from build123d import *

# Parameters (mm, degrees)
F0_W     = 685.8
F0_H     = 101.6
F1_DEPTH = 19.05
F2_W     = 222.25
F2_H     = 14.1
F3_DEPTH = 10.16
F4_R     = 3.302
F5_DEPTH = 25.4


with BuildPart() as f1:
    # F0 (on Front) → F1 (new body)
    with BuildSketch(Plane.XZ):
        with Locations((45.375204, 0)):
            Rectangle(F0_W, F0_H)
    extrude(amount=F1_DEPTH)

    # F2 (on face) → F3 (cut)
    with BuildSketch(Plane(origin=(0, 0, 0), x_dir=(-1, 0, 0), z_dir=(0, 1, 0))):
        with Locations((-258.100204, 0)):
            Rectangle(F2_W, F2_H)
    extrude(amount=-F3_DEPTH, mode=Mode.SUBTRACT)

    # F4 (on face) → F5 (cut)
    with BuildSketch(Plane.XZ.offset(19.05)):
        with BuildLine():
            ThreePointArc((382.052204, 0), (381.085071, 2.334867), (378.750204, 3.302))
            Line((378.750204, 3.302), (378.750204, 0))
            Line((378.750204, 0), (378.750204, -3.302))
            ThreePointArc((378.750204, -3.302), (381.085071, -2.334867), (382.052204, 0))
        make_face()
        with BuildLine():
            Line((378.750204, 0), (378.750204, 3.302))
            ThreePointArc((378.750204, 3.302), (375.448204, 0), (378.750204, -3.302))
            Line((378.750204, -3.302), (378.750204, 0))
        make_face()
        with Locations((137.450204, 0)):
            Circle(F4_R)
        with Locations((-287.999796, 0)):
            Circle(F4_R)
    extrude(amount=-F5_DEPTH, mode=Mode.SUBTRACT)


solid = f1.part
Verification items for the finished model (mm, model axes). Coordinates: 2 decimals unless noted, no trailing zeros. Loops run counter-clockwise (first coordinate to the right, second up) from the corner with the lowest first, then second, coordinate; pieces in that order, holes last. Notation, with made-up numbers: (22.5, 30.25) -> (65.5, 30.25) arc R15 ccw to (65.5, 39.25) -> close; hole circle Ø10 at (2, 67). An arc over 180 degrees is marked (long way). Answer as CSV lines item,"result".
1) Thickness scan on L1, parallel to X at y = -1.25, z = 7; L2, parallel to Z at x = 247.5, y = -5.75; L3, parallel to Y at x = 330, z = -6. Record the ranges inside material, lowest first. Write a range as from..to.
Found:
L1,"x = -297.52..146.98, 369.23..388.28"
L2,"z = -50.8..-7.05, 7.05..50.8"
L3,"y = -19.05..-10.16"
2) Depth check by flat-ended pin: pin 1 (3 mm diameter, centred on x = -108.5, z = -24, fed in from +Y); pin 2 (6 mm diameter, centred on x = 137.45, z = 0, fed in from -Y). Enter the tip coordinate at first touch or a pass-through.
Found:
pin 1,"stops at y = 0"
pin 2,"passes through"
3) Cross-section at B-B, the plane x = 175. Record the cut outline in (y, z), then the cut area to 3 significant figures.
Found:
outline,"(-19.05, -50.8) -> (0, -50.8) -> (0, -7.05) -> (-10.16, -7.05) -> (-10.16, 7.05) -> (0, 7.05) -> (0, 50.8) -> (-19.05, 50.8) -> close"
area,"1,790 mm2"
4) Release check for a two-part mould opening along Z. For faces 1 (the flat face through (260, -10.16, 0)), 2 (the flat face through (41, -9, 50.8)), 3 (the flat face through (41, -9, -50.8)), 4 (the flat face through (41, -19.05, 1)) record: +Z half, -Z half, draft (parallel to the pull), parting line (faces both ways), or undercut.
Found:
face 1,"undercut"
face 2,"+Z half"
face 3,"-Z half"
face 4,"draft"
5) Cross-section at A-A, the plane y = -6.25. Record the cut outline in (x, z).
Found:
outline,"(-297.52, -50.8) -> (388.28, -50.8) -> (388.28, 50.8) -> (-297.52, 50.8) -> close; hole circle Ø6.6 at (-288, 0); hole circle Ø6.6 at (137.45, 0); hole (146.98, -7.05) -> (369.23, -7.05) -> (369.23, 7.05) -> (146.98, 7.05) -> close; hole (378.75, -3.3) arc R3.3 ccw to (382.05, 0) arc R3.3 ccw to (378.75, 3.3) arc R3.3 ccw to start"
